from build123d import *

# Parameters (mm, degrees)
F0_W     = 38.1
F0_H     = 38.1
F1_DEPTH = 711.2
F2_W     = 19.05
F2_H     = 508
F3_DEPTH = 19.05
F4_W     = 31.75
F4_H     = 31.75
F5_DEPTH = 711.201


with BuildPart() as f1:
    # F0 (on Top) → F1 (new body)
    with BuildSketch(Plane.XY):
        with Locations((19.05, 19.05)):
            Rectangle(F0_W, F0_H)
    extrude(amount=F1_DEPTH)

    # F2 (on face) → F3 (cut)
    with BuildSketch(Plane.XZ):
        with Locations((28.575, 457.2)):
            Rectangle(F2_W, F2_H)
    extrude(amount=-F3_DEPTH, mode=Mode.SUBTRACT)

    # F4 (on face) → F5 (cut, through all)
    with BuildSketch(Plane(origin=(0, 0, 0), x_dir=(1, 0, 0), z_dir=(0, 0, -1))):
        with Locations((19.05, -19.05)):
            Rectangle(F4_W, F4_H)
    extrude(amount=-F5_DEPTH, mode=Mode.SUBTRACT)


solid = f1.part
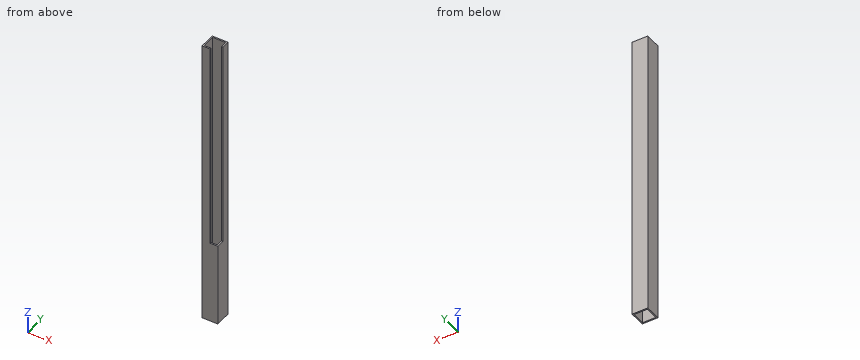
Input: part model. Units: mm. Frame: model coordinates. Coordinates: 2 decimals unless noted, no trailing zeros. Loops run counter-clockwise (first coordinate to the right, second up) from the corner with the lowest first, then second, coordinate; pieces in that order, holes last. Notation, with made-up numbers: (79, -39.5) - (131, -39.5) arc R13 cw to (131, -23.5) - close; hole circle Ø5 at (5.5, 34.25). An arc over 180 degrees is marked (long way). Answer in a Markdown table with one row per item. Add a question column.
Item 1: Contact query for flat-ended pins moving along their axis: P1, Ø3.5, axis at y = 1.5, z = 495.5, coming from the +X side; P2, Ø3.5, axis at x = 35.5, z = 385, coming from the -Y side; P3, Ø2, axis at x = 20, z = 408, coming from the -Y side; P4, Ø15, axis at x = 33.5, y = 10.5, coming from the +Z side. Output: stop coordinate, or through.
Item 2: Section query A-A on x = 13. Return the cut outline in (y, z) (3 decimals), then the cut area to 3 significant figures.
Item 3: Line query: line 1 along Y through (x, z) = (16.5, 367) (3 decimals); line 2 along X through (y, z) = (2.5, 284). Output: solid intervals per line, ascending. Write a range as [from, to].
Item 4: Section query C-C on z = 406.5. Return the cut outline in (x, y) (3 decimals).
Item 5: Section query B-B on z = 176.5. Return the cut outline in (x, y) (3 decimals).
Recorded:
| question | item | result |
|---|---|---|
| 1 | P1 | x = 19.05 |
| 1 | P2 | y = 19.05 |
| 1 | P3 | y = 0 |
| 1 | P4 | z = 203.2 |
| 2 | outline | (0, 0) - (3.175, 0) - (3.175, 711.2) - (0, 711.2) - close; (34.925, 0) - (38.1, 0) - (38.1, 711.2) - (34.925, 711.2) - close |
| 2 | area | 4,520 mm^2 |
| 3 | line 1 | [0, 3.175], [34.925, 38.1] |
| 3 | line 2 | [0, 19.05] |
| 4 | outline | (0, 0) - (19.05, 0) - (19.05, 3.175) - (3.175, 3.175) - (3.175, 34.925) - (34.925, 34.925) - (34.925, 19.05) - (38.1, 19.05) - (38.1, 38.1) - (0, 38.1) - close |
| 5 | outline | (0, 0) - (38.1, 0) - (38.1, 38.1) - (0, 38.1) - close; hole (3.175, 3.175) - (34.925, 3.175) - (34.925, 34.925) - (3.175, 34.925) - close |
